from build123d import *

# Parameters (mm, degrees)
SKETCH1_W           = 125
SKETCH1_H           = 125
BOSS_EXTRUDE1_DEPTH = 4
SKETCH7_W           = 40
SKETCH7_H           = 69.5
BOSS_EXTRUDE4_DEPTH = 4
SKETCH8_W           = 69.5
SKETCH8_H           = 30
BOSS_EXTRUDE5_DEPTH = 4
BOSS_EXTRUDE2_DEPTH = 10
SKETCH3_R           = 10
BOSS_EXTRUDE3_DEPTH = 4
SKETCH4_R           = 5.25
CUT_EXTRUDE1_DEPTH  = 4
FILLET1_R           = 125
CHAMFER1_SIZE       = 5
CHAMFER1_SIZE2      = 8.660254038
BOSS_EXTRUDE6_DEPTH = 14
FILLET2_R           = 10


with BuildPart() as part:
    # Sketch1 → Boss-Extrude1 (new body)
    with BuildSketch(Plane(origin=(0, 0, 0), x_dir=(1, 0, 0), z_dir=(0, 1, 0))):
        Rectangle(SKETCH1_W, SKETCH1_H)
    extrude(amount=BOSS_EXTRUDE1_DEPTH)

    # Sketch7 → Boss-Extrude4 (add)
    with BuildSketch(Plane(origin=(0, 0, 0), x_dir=(1, 0, 0), z_dir=(0, 1, 0))):
        with Locations((82.5, 27.75)):
            Rectangle(SKETCH7_W, SKETCH7_H)
    extrude(amount=BOSS_EXTRUDE4_DEPTH)

    # Sketch8 → Boss-Extrude5 (add)
    with BuildSketch(Plane(origin=(0, 0, 0), x_dir=(1, 0, 0), z_dir=(0, 1, 0))):
        with Locations((-27.75, -77.5)):
            Rectangle(SKETCH8_W, SKETCH8_H)
    extrude(amount=BOSS_EXTRUDE5_DEPTH)

    # Sketch2 → Boss-Extrude2 (add)
    with BuildSketch(Plane(origin=(0, 4, 0), x_dir=(1, 0, 0), z_dir=(0, 1, 0))):
        with BuildLine():
            Line((-62.5, -92.5), (-62.5, 62.5))
            Line((-62.5, 62.5), (102.5, 62.5))
            Line((102.5, 62.5), (102.5, 54))
            Line((102.5, 54), (62.5, 54))
            ThreePointArc((62.5, 54), (-19.877940008, 19.877940008), (-54, -62.5))
            Line((-54, -62.5), (-54, -92.5))
            Line((-54, -92.5), (-62.5, -92.5))
        make_face()
    extrude(amount=BOSS_EXTRUDE2_DEPTH)

    # Sketch3 → Boss-Extrude3 (add)
    with BuildSketch(Plane(origin=(0, 4, 0), x_dir=(1, 0, 0), z_dir=(0, 1, 0))):
        with Locations((62.5, -62.5)):
            Circle(SKETCH3_R)
    extrude(amount=-BOSS_EXTRUDE3_DEPTH)

    # Sketch4 → Cut-Extrude1 (cut)
    with BuildSketch(Plane(origin=(0, 4, 0), x_dir=(1, 0, 0), z_dir=(0, 1, 0))):
        with Locations(Location((62.5, -62.5, 0), (0, 0, 270))):
            Circle(SKETCH4_R)
    extrude(amount=-CUT_EXTRUDE1_DEPTH, mode=Mode.SUBTRACT)

    # Fillet1
    fillet1_edges = [part.edges().sort_by_distance(p)[0] for p in [
        (-62.5, 7, -62.5),
    ]]
    fillet(fillet1_edges, radius=FILLET1_R)

    # Chamfer1
    chamfer1_edges = [part.edges().sort_by_distance(p)[0] for p in [
        (102.5, 9, -54),
    ]]
    chamfer1_side = [part.faces().sort_by_distance(p)[0] for p in [
        (102.5, 3.639118457, -34.891873278),
    ]]
    chamfer(chamfer1_edges, length=CHAMFER1_SIZE, length2=CHAMFER1_SIZE2, reference=chamfer1_side[0])

    # Sketch9 → Boss-Extrude6 (add)
    with BuildSketch(Plane(origin=(0, 0, 0), x_dir=(1, 0, 0), z_dir=(0, 1, 0))):
        with BuildLine():
            Line((102.5, -7), (102.5, -21.193220895))
            ThreePointArc((102.5, -21.193220895), (90.917033755, -12.512779707), (77.533296378, -7))
            Line((77.533296378, -7), (102.5, -7))
        make_face()
    extrude(amount=BOSS_EXTRUDE6_DEPTH)

    # Fillet2
    fillet2_edges = [part.edges().sort_by_distance(p)[0] for p in [
        (62.5, 2, 7),
        (7, 2, 62.5),
        (62.5, 2, 52.5),
        (52.5, 2, 62.5),
    ]]
    fillet(fillet2_edges, radius=FILLET2_R)


solid = part.part
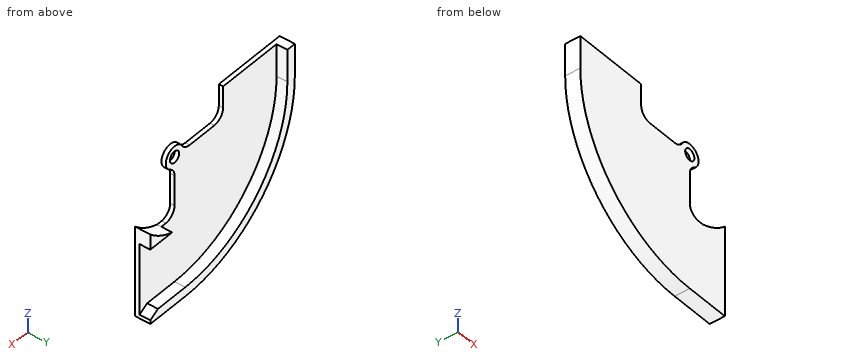
Verification items for the finished model (mm, model axes). Coordinates: 2 decimals unless noted, no trailing zeros. Order: outer loops, then holes, each group sorted by start corner. A loop starts at its lowest first (then second) coordinate and runs counter-clockwise, first axis right, second up.
Item 1: Section check C-C, the plane z = -17. Enter the section's corners in (x, y), then the cut area to 3 significant figures.
Filled in:
outline: (-33.96, 0) - (102.5, 0) - (102.5, 4) - (-22.66, 4) - (-22.66, 14) - (-33.96, 14) - close
area: 659 mm2
Item 2: Section check A-A, the plane y = 11.75. Enter the section's corners in (x, z).
Filled in:
outline: (-62.5, 62.5) arc R125 ccw to (62.5, -62.5) - (102.5, -62.5) - (102.5, -59) - (93.84, -54) - (62.5, -54) arc R116.5 cw to (-54, 62.5) - (-54, 92.5) - (-62.5, 92.5) - close; (77.53, 7) - (102.5, 7) - (102.5, 21.19) arc R57.5 cw to start
Item 3: Section check B-B, the plane x = 81.5. Enter the section's corners in (y, z), then the cut area to 3 significant figures.
Filled in:
outline: (0, -62.5) - (14, -62.5) - (14, -54) - (4, -54) - (4, 7) - (14, 7) - (14, 8.23) - (0, 8.23) - close
area: 380 mm2
Item 4: Depth check by flat-ended pin: pin 1 (2 mm diameter, centred on x = 16, y = 9.5, fed in from +Z); pin 2 (4.5 mm diameter, centred on x = 74, y = 3, fed in from +Z); pin 3 (6 mm diameter, centred on y = 7, z = 40.5, fed in from -X); pin 4 (12 mm diameter, centred on x = 62.5, z = 62.5, fed in from -Y). Enter the tip coordinate at first touch or a pass-through.
Filled in:
pin 1: stops at z = -43.88
pin 2: stops at z = 66.3
pin 3: stops at x = -61.05
pin 4: stops at y = 0
Item 5: Material ranges on L1, parallel to Y at x = 24.5, z = -14.5; L2, parallel to X at y = 5.25, z = 78; L3, parallel to X at y = 1, z = 83, recorded low to high.
Filled in:
L1: y = 0 to 4
L2: x = -62.5 to -54
L3: x = -62.5 to 7
Item 6: Section check D-D, the plane x = -7. Enter the section's corners in (y, z), then the cut area to 3 significant figures.
Filled in:
outline: (0, -41.4) - (14, -41.4) - (14, -31) - (4, -31) - (4, 92.5) - (0, 92.5) - close
area: 640 mm2
